Geometry: final body of the model. Coordinates: model frame, mm. Face numbers are marked on the shaded views. A direction names the side the tool comes from. Round coordinates to 2 decimals unless told otherwise and drop trailing zeros. Write each loop counter-clockwise with the first axis right and the second up, starting at its lowest first coordinate (ties: lowest second). Pieces come first, ordered by that corner, then holes. Notation, with made-up numbers: (-16, 48.25) - (32, 48.25) arc R13 cw to (32, 55.25) - close; hole circle Ø9 at (-2.5, -40). An arc over 180 degrees is marked (long way). Write each question's results on one line, items separated by ' | '.
from build123d import *

# Parameters (mm, degrees)
BOSS_EXTRUDE1_DEPTH  = 84.455
BOSS_EXTRUDE2_DEPTH  = 5
FILLET2_R            = 15
CUT_EXTRUDE1_DEPTH   = 4
FILLET2_OF_MIRROR1_R = 15
FILLET1_START        = -79.455
FILLET1_DEPTH        = 158.91


with BuildPart() as part:
    # Sketch1 → Boss-Extrude1 (new, symmetric)
    with BuildSketch(Plane(origin=(0, 0, 0), x_dir=(0, 0, -1), z_dir=(1, 0, 0))):
        Polygon((0, 63.5), (0, 0), (68.9125, 0), (4, 4), align=None)
    extrude(amount=BOSS_EXTRUDE1_DEPTH, both=True)

    # Sketch2 → Boss-Extrude2 (add)
    with BuildSketch(Plane(origin=(84.455, 0, 0), x_dir=(0, 0, -1), z_dir=(1, 0, 0))):
        Polygon((0, 63.5), (24.219826303, 25.26657899), (61.769719172, 0), (0, 0), align=None)
    boss_extrude2 = extrude(amount=-BOSS_EXTRUDE2_DEPTH)

    # Fillet2
    fillet2_edges = [part.edges().sort_by_distance(p)[0] for p in [
        (79.455, 33.75, -2),
    ]]
    fillet(fillet2_edges, radius=FILLET2_R)

    # Sketch4 → Cut-Extrude1 (cut)
    with BuildSketch(Plane(origin=(84.455, 0, 0), x_dir=(0, 0, -1), z_dir=(1, 0, 0))):
        Polygon((0, 19), (20, 19), (25, 14), (20, 9), (0, 9), align=None)
    cut_extrude1 = extrude(amount=-CUT_EXTRUDE1_DEPTH, mode=Mode.SUBTRACT)

    # Mirror1: Boss-Extrude2, Cut-Extrude1 across plane
    add(boss_extrude2.mirror(Plane(origin=(0, 0, 0), x_dir=(0, 0, 1), z_dir=(1, 0, 0))))
    add(cut_extrude1.mirror(Plane(origin=(0, 0, 0), x_dir=(0, 0, 1), z_dir=(1, 0, 0))), mode=Mode.SUBTRACT)

    # Fillet2 of Mirror1
    fillet2_of_mirror1_edges = [part.edges().sort_by_distance(p)[0] for p in [
        (-79.455, 33.75, -2),
    ]]
    fillet(fillet2_of_mirror1_edges, radius=FILLET2_OF_MIRROR1_R)

    # Fillet1: read off the stored shape, not the designer's step
    # Fillet1 outline → Fillet1 (add)
    with BuildSketch(Plane.YZ.offset(FILLET1_START)):
        with BuildLine():
            Line((4, -4), (3.038172839, -19.608651391))
            add(Edge.make_bspline(
                [(3.038172839, -19.608651391), (4, -4), (36.630400727, -1.806359615)],
                knots=[0, 0, 0, 1, 1, 1], degree=2, weights=[1, 0.7511041, 1]))
            Line((36.630400727, -1.806359615), (4, -4))
        make_face()
    extrude(amount=FILLET1_DEPTH)


solid = part.part
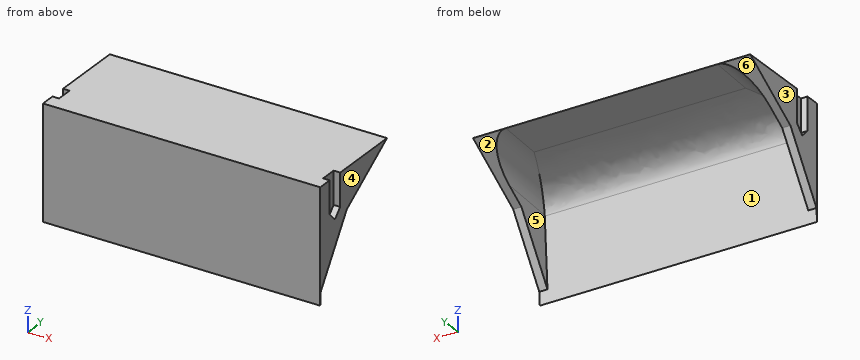
Q1. Mould query, pull axis X, two halves, no side actions, for the marked faces 1, 2, 3 and 4. Classes: pulls with the +X half, pulls with the -X half, needs draft (parallel to the pull), parting line crosses it, or undercut.
Answer block:
face 1: undercut | face 2: needs draft | face 3: pulls with the -X half | face 4: pulls with the +X half
Q2. Pin query (flat end, axial travel): pin 1 (2 mm diameter, centred on x = 17, z = -37, fed in from -Y); pin 2 (12 mm diameter, centred on x = 59, z = -17, fed in from +Y); pin 3 (8 mm diameter, centred on x = 17.5, y = 20, fed in from -Z); pin 4 (8 mm diameter, centred on x = -34, y = 22, fed in from -Z). Return the tip coordinate at first contact, or that it passes through.
Answer block:
pin 1: y = 0 | pin 2: y = 8.21 | pin 3: z = -6.42 | pin 4: z = -5.62
Q3. Ray query, line 1 along X through (y, z) = (18, -18) (3 decimals); line 2 along Z through (x, y) = (-15.5, 19); line 3 along Z through (x, y) = (-5, 10.5). Return the intervals inside material, ascending.
Answer block:
line 1: -80.455 to -79.455, 79.455 to 80.455 | line 2: -5.25 to 0 | line 3: -9.32 to 0
Q4. Access query for the marked faces 5 and 6. Directions: +Z, -Z, +X, -X, +Y, -Y. A direction counts if a zero-diameter tool reaches every point of the face in a straight line with its end or side. Return the directions, or none.
Answer block:
face 5: -Z, +Y | face 6: -Z, +X, -X, +Y
Q5. Section query A-A, the plane z = -47. Return loops of the section in (x, y) (3 decimals).
Answer block:
outline: (-84.455, 0) - (84.455, 0) - (84.455, 9.938) - (79.455, 9.938) - (79.455, 1.35) - (-79.455, 1.35) - (-79.455, 9.938) - (-84.455, 9.938) - close
Q6. Section query B-B, the plane z = -58.5. Return loops of the section in (x, y) (3 decimals), plus the area to 3 significant figures.
Answer block:
outline: (-84.455, 0) - (84.455, 0) - (84.455, 2.2) - (79.455, 2.2) - (79.455, 0.642) - (-79.455, 0.642) - (-79.455, 2.2) - (-84.455, 2.2) - close | area: 124 mm2
